Source: CAD feature listing. Evaluate the final solid. Frame: model axes, mm. A direction names the side the tool comes from. Give positions to 0.01 mm unless a question says otherwise; leave off trailing zeros. Loops run counter-clockwise (first coordinate to the right, second up) from the corner with the lowest first, then second, coordinate; pieces in that order, holes last. Notation, with made-up numbers: (-20.75, 60) -> (21.25, 60) arc R26 cw to (21.25, 99) -> close; hole circle Ø1 at (-14, -26.5). An arc over 180 degrees is marked (long way). Put each result on its own line as item: value.
```python
from build123d import *

# Parameters (mm, degrees)
SKETCH1_W           = 5
SKETCH1_H           = 20
BOSS_EXTRUDE1_DEPTH = 5


with BuildPart() as part:
    # Sketch1 → Boss-Extrude1 (new body)
    with BuildSketch(Plane.XY):
        Polygon((-70, 20), (-59.5, 20), (-59.5, 25), (-44.5, 25), (-44.5, 20), (-29.5, 20), (-29.5, 25), (-14.5, 25), (-14.5, 20), (14.5, 20), (14.5, 25), (29.5, 25), (29.5, 20), (44.5, 20), (44.5, 25), (59.5, 25), (59.5, 20), (70, 20), (70, 10), (75, 10), (75, -10), (70, -10), (70, -20), (59.5, -20), (59.5, -25), (44.5, -25), (44.5, -20), (29.5, -20), (29.5, -25), (14.5, -25), (14.5, -20), (-14.5, -20), (-14.5, -25), (-29.5, -25), (-29.5, -20), (-44.5, -20), (-44.5, -25), (-59.5, -25), (-59.5, -20), (-70, -20), (-70, -10), (-75, -10), (-75, 10), (-70, 10), align=None)
        with Locations((35, 0)):
            Rectangle(SKETCH1_W, SKETCH1_H, mode=Mode.SUBTRACT)
        Rectangle(SKETCH1_W, SKETCH1_H, mode=Mode.SUBTRACT)
        with Locations((-35, 0)):
            Rectangle(SKETCH1_W, SKETCH1_H, mode=Mode.SUBTRACT)
    extrude(amount=BOSS_EXTRUDE1_DEPTH)


solid = part.part
```
(1) Reachability of faces 1 (the flat face through (44.5, 22, 2)), 2 (the flat face through (-59.5, 22, 2)), 3 (the flat face through (44.5, -23, 2)) from +Z, -Z, +X, -X, +Y, -Y: full face, straight path, thin tool, end or side. Return the list, or none.
Calculated:
face 1: +Z, -Z, +Y
face 2: +Z, -Z, -X, +Y
face 3: +Z, -Z, -Y
(2) Draft query along X for faces 4 (the flat face through (70, -15, 2)), 5 (the flat face through (0, -10, 2)), 6 (the flat face through (-52, 25, 2)). Return one class per face: released by +X, released by -X, zero draft, split by the parting line, or undercut.
Calculated:
face 4: released by +X
face 5: undercut
face 6: zero draft
(3) First-contact query: P1, Ø1.5, axis at x = -72.5, z = 3.5, coming from the +Y side; P2, Ø2.5, axis at y = -22.5, z = 2.5, coming from the +X side; P3, Ø2, axis at x = -29, y = 14, coming from the -Z side; P4, Ø1.5, axis at x = 34.5, z = 2.5, coming from the +Y side. Flat tips, straight axial feed; report the tip coordinate or a pass-through.
Calculated:
P1: stops at y = 10
P2: stops at x = 59.5
P3: stops at z = 0
P4: stops at y = 20
(4) Section C-C on z = 4.15. Give the number of separate pieces and of enclosed holes in the cut face, then the cut area to 3 significant figures.
Calculated:
separate pieces: 1
enclosed holes: 3
area: 6,100 mm²
(5) Line query: probe 1 along X at (y, z) = (21.5, 2.3); probe 2 along X at (y, z) = (-8.5, 2.35); probe 3 along Y at (x, z) = (37, 1.95). Output: solid intervals per line, ascending. Write a range as from..to.
Calculated:
probe 1: x = -59.5..-44.5, -29.5..-14.5, 14.5..29.5, 44.5..59.5
probe 2: x = -75..-37.5, -32.5..-2.5, 2.5..32.5, 37.5..75
probe 3: y = -20..-10, 10..20
(6) Section B-B on x = 36. Return loops of the section in (y, z).
Calculated:
outline: (-20, 0) -> (-10, 0) -> (-10, 5) -> (-20, 5) -> close; (10, 0) -> (20, 0) -> (20, 5) -> (10, 5) -> close
(7) Section A-A on y = 5.5. Return loops of the section in (x, z).
Calculated:
outline: (-75, 0) -> (-37.5, 0) -> (-37.5, 5) -> (-75, 5) -> close; (-32.5, 0) -> (-2.5, 0) -> (-2.5, 5) -> (-32.5, 5) -> close; (2.5, 0) -> (32.5, 0) -> (32.5, 5) -> (2.5, 5) -> close; (37.5, 0) -> (75, 0) -> (75, 5) -> (37.5, 5) -> close
(8) Section D-D on x = -42. Return loops of the section in (y, z).
Calculated:
outline: (-20, 0) -> (20, 0) -> (20, 5) -> (-20, 5) -> close
